from build123d import *

# Parameters (mm, degrees)
F1_DEPTH = 30
F2_SIZE  = 5.08
F3_R     = 5.08


with BuildPart() as f1:
    # F0 (on Front) → F1 (new body)
    with BuildSketch(Plane.XZ):
        Polygon((-72.913893, 47.520347), (-72.913893, 43.428164), (-11.468264, 29.078148), (16.188771, 75.537905), (-61.714064, 52.23044), align=None)
    extrude(amount=F1_DEPTH)

    # F2
    f2_edges = [f1.edges().sort_by_distance(p)[0] for p in [
        (-22.762647, -30, 63.884173),
    ]]
    chamfer(f2_edges, length=F2_SIZE)

    # F3
    f3_edges = [f1.edges().sort_by_distance(p)[0] for p in [
        (16.188771, -12.46, 75.537905),
    ]]
    fillet(f3_edges, radius=F3_R)


solid = f1.part
Design review of the part built by this model. Coordinates are the model's own, in mm. Coordinates: 2 decimals unless noted, no trailing zeros. Order: outer loops, then holes, each group sorted by start corner. A loop starts at its lowest first (then second) coordinate and runs counter-clockwise, first axis right, second up. Notation, with made-up numbers: M 19,3 L 75,3 A17 ccw 75,9 Z; hole C -1.5,84.25 d1. An arc over 180 degrees is marked long. Use a Markdown table: item, result.
(1) Wall thickness on probe 1 along Z at (x, y) = (-28.5, -3); probe 2 along X at (y, z) = (-5, 49); probe 3 along Z at (x, y) = (-69, -24.5): over which ranges is each line inside the solid? List them lowest first.
Worked answers:
| item | result |
|---|---|
| probe 1 | z = 33.06 to 62.17 |
| probe 2 | x = -69.4 to 0.39 |
| probe 3 | z = 42.51 to 49.17 |
(2) Add section D-D (z = 32). Give the boundary of the cut face in (x, y), then the cut area to 3 significant figures.
Worked answers:
| item | result |
|---|---|
| outline | M -23.98,-30 L -9.73,-30 L -9.73,0 L -23.98,0 Z |
| area | 428 mm2 |
(3) For P1, Ø5, axis at x = -13.5, z = 64.5, coming from the +Y side; P2, Ø1, axis at x = -54, y = -4, coming from the -Z side; P3, Ø4, axis at x = -16, y = -10.5, coming from the +Z side; P4, Ø5, axis at x = 1, y = -19.5, coming from the +Z side, all flat-tipped, find the tip position at first contact; note any pin that passes through.
Worked answers:
| item | result |
|---|---|
| P1 | stops at y = 0 |
| P2 | stops at z = 38.89 |
| P3 | stops at z = 66.51 |
| P4 | stops at z = 71.74 |
(4) Add section A-A (y = -7). Give the boundary of the cut face in (x, z).
Worked answers:
| item | result |
|---|---|
| outline | M -72.91,43.43 L -11.47,29.08 L 9.52,64.34 A5.08 ccw 3.7,71.8 L -61.71,52.23 L -72.91,47.52 Z |
(5) Add section B-B (x = 5). Give the boundary of the cut face in (y, z), then the cut area to 3 significant figures.
Worked answers:
| item | result |
|---|---|
| outline | M -30,56.74 L 0,56.74 L 0,72.01 L -25.09,72.01 L -30,66.89 Z |
| area | 446 mm2 |
(6) Add section C-C (z = 60.5). Give the boundary of the cut face in (x, y), then the cut area to 3 significant figures.
Worked answers:
| item | result |
|---|---|
| outline | M -34.07,-24.92 L -16.35,-30 L 7.24,-30 L 7.24,0 L -34.07,0 Z |
| area | 1,190 mm2 |
